Could you check a few things on this model? Use its own coordinates, in mm. Give positions to 0.01 mm unless a question says otherwise; leave off trailing zeros. Loops run counter-clockwise (first coordinate to the right, second up) from the corner with the lowest first, then second, coordinate; pieces in that order, holes last. Notation, with made-up numbers: (-31, 89.25) -> (20, 89.25) arc R27 cw to (20, 106.25) -> close; hole circle Ø10 at (18, 79.25). An arc over 180 degrees is marked (long way). Write each question's results on one line, items separated by ' | '. Start each with the question number.
Q1. If I drill on line 1 along Y through (x, z) = (2, -135.5); line 2 along Y through (x, z) = (-2.5, 0.5); line 3 along Z through (x, y) = (4.5, -926.5), over which ranges is the centre line in solid material (lowest first)?
Q2. Will these pins go through, and if not, where does the flat tip stop? P1, Ø6.5, axis at x = 2, y = -404, coming from the +Z side; P2, Ø4, axis at x = -3, z = 111.5, coming from the -Y side; P3, Ø5, axis at x = 1, y = -508.5, coming from the -Z side.
Q3. If we section it at B-B, the plane x = 0: List the corners of the cut face in (y, z) for me, plus the area to 3 significant figures.
Q4. If we section it at A-A, the plane z = -142.5: List the corners of the cut face in (x, y) for me.
Q5. If we section it at C-C, the plane y = -89: List the corners of the cut face in (x, z) for me.
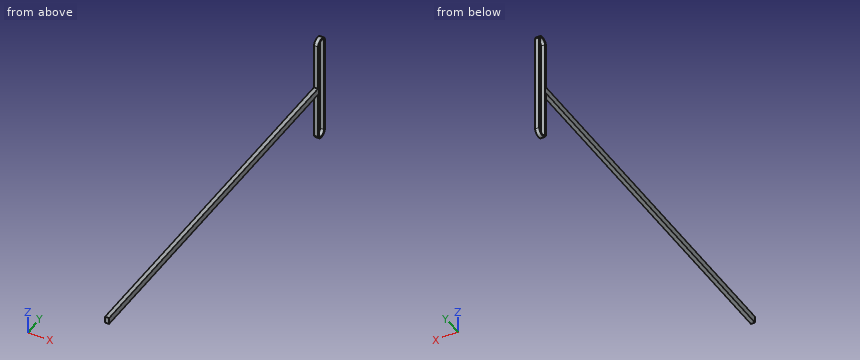
from build123d import *

# Parameters (mm, degrees)
BOSS_EXTRUDE1_DEPTH = 6.5
SKETCH3_W           = 13
SKETCH3_H           = 20.987716218
BOSS_EXTRUDE2_DEPTH = 1200


with BuildPart() as part:
    # Sketch1 → Boss-Extrude1 (new, symmetric)
    with BuildSketch(Plane(origin=(0, 0, 0), x_dir=(0, 0, -1), z_dir=(1, 0, 0))):
        with BuildLine():
            Line((-160.579938889, -20), (160.579938889, -20))
            ThreePointArc((160.579938889, -20), (176.670722942, 0), (160.579938889, 20))
            Line((160.579938889, 20), (-160.579938889, 20))
            ThreePointArc((-160.579938889, 20), (-176.670722942, 0), (-160.579938889, -20))
        make_face()
        with BuildLine():
            Line((-160, 15), (160, 15))
            ThreePointArc((160, 15), (171.670722942, 0), (160, -15))
            Line((160, -15), (-160, -15))
            ThreePointArc((-160, -15), (-171.670722942, 0), (-160, 15))
        make_face(mode=Mode.SUBTRACT)
    extrude(amount=BOSS_EXTRUDE1_DEPTH, both=True)

    # Sketch3 → Boss-Extrude2 (add)
    with BuildSketch(Plane.XZ.offset(20)):
        Rectangle(SKETCH3_W, SKETCH3_H)
    extrude(amount=BOSS_EXTRUDE2_DEPTH)


solid = part.part
Final values:
1) line 1: y = -20 to -15, 15 to 20 | line 2: y = -1220 to -15, 15 to 20 | line 3: z = -10.49 to 10.49
2) P1: stops at z = 10.49 | P2: stops at y = -20 | P3: stops at z = -10.49
3) outline: (-1220, -10.49) -> (-20, -10.49) -> (-20, -160.58) arc R20.47 ccw to (20, -160.58) -> (20, 160.58) arc R20.47 ccw to (-20, 160.58) -> (-20, 10.49) -> (-1220, 10.49) -> close; hole (-15, -160) arc R15.47 ccw to (15, -160) -> (15, 160) arc R15.47 ccw to (-15, 160) -> close | area: 28,900 mm²
4) outline: (-6.5, -20) -> (6.5, -20) -> (6.5, -15) -> (-6.5, -15) -> close; (-6.5, 15) -> (6.5, 15) -> (6.5, 20) -> (-6.5, 20) -> close
5) outline: (-6.5, -10.49) -> (6.5, -10.49) -> (6.5, 10.49) -> (-6.5, 10.49) -> close
